from build123d import *

# Parameters (mm, degrees)
EXTRUDE_1_DEPTH     = 1
CUT_EXTRUDE_1_DEPTH = 1


with BuildPart() as part:
    # 草图1 → 凸台-拉伸1 (new body)
    with BuildSketch(Plane(origin=(0, 0, 0), x_dir=(1, 0, 0), z_dir=(0, 1, 0))):
        Polygon((-27, 30), (-30, 27), (-30, 3), (-27, 0), (-3, 0), (0, 3), (0, 27), (-3, 30), align=None)
    extrude(amount=EXTRUDE_1_DEPTH)

    # 草图2 → 切除-拉伸1 (cut)
    with BuildSketch(Plane(origin=(0, 0, 0), x_dir=(1, 0, 0), z_dir=(0, 1, 0))):
        Polygon((-26.768491702, 25.375210501), (-27.571851102, 24.571851102), (-23.608439528, 20.608439528), (-22.805080129, 21.411798927), align=None)
        Polygon((-3.231508298, 25.375210501), (-2.428148898, 24.571851102), (-6.391560472, 20.608439528), (-7.194919871, 21.411798927), align=None)
        Polygon((-25.835128567, 2.771590231), (-25.031769168, 1.968230832), (-21.433586648, 5.566413352), (-22.236946047, 6.369772752), align=None)
        Polygon((-4.968230832, 1.968230832), (-4.164871433, 2.771590231), (-7.763215817, 6.369934615), (-8.566575216, 5.566575216), align=None)
    extrude(amount=CUT_EXTRUDE_1_DEPTH, mode=Mode.SUBTRACT)


solid = part.part
Could you check a few things on this model? Use its own coordinates, in mm. A direction names the side the tool comes from. Coordinates: 2 decimals unless noted, no trailing zeros. Order: outer loops, then holes, each group sorted by start corner. A loop starts at its lowest first (then second) coordinate and runs counter-clockwise, first axis right, second up. Notation, with made-up numbers: (-3, 3.25) - (27, 3.25) arc R15 cw to (27, 12.25) - close; hole circle Ø8 at (1.25, 33). An arc over 180 degrees is marked (long way). Answer in a Markdown table with one row per item. Add a question column.
(1) If we section it at A-A, the plane y = 0.45: Please give me the cut outline in (x, z).
(2) On a 3-axis mill with a long thin cutter (end or side, diameter ignored), from which of +Z, -Z, +X, -X, +Y, -Y can I reach the whole of each face in a straight line? I mean faces 1 (the face through (-6.788, 0.493, -21.004)), 2 (the face through (-15, 1, -15)). Say none if no direction works.
(3) Will this pin go through, and if not, where does the flat tip stop? pin 1 (8 mm diameter, centred on x = -7, z = -16, fed in from -Y).
(4) I need wall thicknesses on L1, parallel to Z at x = -24.25, y = 0.1; L2, parallel to Z at x = -7, y = 0.65; L3, parallel to X at y = 0.8, z = -4.75. Which ranges of each line are inside material? Lowest first, please.
(5) If we section it at C-C, the plane z = -28: Please give me the cut outline in (x, y).
(6) If we section it at B-B, the plane x = -6: Please give me the cut outline in (y, z).
(7) If we mould it in two halves opening along Z, with no side actions, what happens to faces 3 (the face through (0, 0.5, -14.8)), 4 (the face through (-1.5, 0.5, -1.5)), 5 (the face through (-1.5, 0.5, -28.5)), 6 (the face through (-4.4, 0.5, -22.6))? For each: released by +Z, released by -Z, zero draft, split by the parting line, or undercut.
Results are:
| question | item | result |
|---|---|---|
| 1 | outline | (-30, -27) - (-27, -30) - (-3, -30) - (0, -27) - (0, -3) - (-3, 0) - (-27, 0) - (-30, -3) - close; hole (-27.57, -24.57) - (-26.77, -25.38) - (-22.81, -21.41) - (-23.61, -20.61) - close; hole (-25.84, -2.77) - (-22.24, -6.37) - (-21.43, -5.57) - (-25.03, -1.97) - close; hole (-8.57, -5.57) - (-7.76, -6.37) - (-4.16, -2.77) - (-4.97, -1.97) - close; hole (-7.19, -21.41) - (-3.23, -25.38) - (-2.43, -24.57) - (-6.39, -20.61) - close |
| 2 | face 1 | +Y, -Y |
| 2 | face 2 | +Z, -Z, +X, -X, +Y |
| 3 | pin 1 | stops at y = 0 |
| 4 | L1 | z = -30 to -22.86, -21.25 to -4.36, -2.75 to 0 |
| 4 | L2 | z = -30 to -21.61, -21.22 to -5.61, -4 to 0 |
| 4 | L3 | x = -30 to -23.86, -22.25 to -7.75, -6.14 to 0 |
| 5 | outline | (-29, 0) - (-1, 0) - (-1, 1) - (-29, 1) - close |
| 6 | outline | (0, -30) - (1, -30) - (1, -22.61) - (0, -22.61) - close; (0, -21) - (1, -21) - (1, -4.61) - (0, -4.61) - close; (0, -3) - (1, -3) - (1, 0) - (0, 0) - close |
| 7 | face 3 | zero draft |
| 7 | face 4 | released by +Z |
| 7 | face 5 | released by -Z |
| 7 | face 6 | undercut |
